from build123d import *

# Parameters (mm, degrees)
EXTRUDE_1_DEPTH             = 40
CUT_EXTRUDE_2_REACH         = 89.321
HOLE_WIZARD_M5_1_AT_2_COUNT = 2
HOLE_WIZARD_M5_1_AT_2_PITCH = 66.468037432
HOLE_WIZARD_M5_1_AT_3_COUNT = 2
HOLE_WIZARD_M5_1_AT_3_PITCH = 94
HOLE_WIZARD_M5_1_AT_4_COUNT = 2
HOLE_WIZARD_M5_1_AT_4_PITCH = 66.468037432
SKETCH_5_R                  = 17.5
CUT_EXTRUDE_3_DEPTH         = 10


with BuildPart() as part:
    # 草图1 → 拉伸1 (new, symmetric)
    with BuildSketch(Plane.XY):
        Polygon((-20, 0), (10, 0), (10, 85), (0, 85), (0, 10), (-20, 10), align=None)
    extrude(amount=EXTRUDE_1_DEPTH, both=True)

    # 草图2 → 拉伸2 (cut, up to next)
    with BuildSketch(Plane(origin=(0, 10, 0), x_dir=(1, 0, 0), z_dir=(0, 1, 0)), mode=Mode.PRIVATE) as cut_extrude_2_sk1:
        with BuildLine():
            Line((-13.5, 25), (-13.5, 15))
            ThreePointArc((-13.5, 15), (-10, 11.5), (-6.5, 15))
            Line((-6.5, 15), (-6.5, 25))
            ThreePointArc((-6.5, 25), (-10, 28.5), (-13.5, 25))
        make_face()
    cut_extrude_2_tool1 = extrude(cut_extrude_2_sk1.sketch, amount=-CUT_EXTRUDE_2_REACH, mode=Mode.PRIVATE) & part.part
    # 草图2 → 拉伸2 (cut, up to next)
    with BuildSketch(Plane(origin=(0, 10, 0), x_dir=(1, 0, 0), z_dir=(0, 1, 0)), mode=Mode.PRIVATE) as cut_extrude_2_sk2:
        with BuildLine():
            Line((-13.5, -15), (-13.5, -25))
            ThreePointArc((-13.5, -25), (-10, -28.5), (-6.5, -25))
            Line((-6.5, -25), (-6.5, -15))
            ThreePointArc((-6.5, -15), (-10, -11.5), (-13.5, -15))
        make_face()
    cut_extrude_2_tool2 = extrude(cut_extrude_2_sk2.sketch, amount=-CUT_EXTRUDE_2_REACH, mode=Mode.PRIVATE) & part.part
    add(cut_extrude_2_tool1.solids().sort_by_distance((-10, 10, -20))[0], mode=Mode.SUBTRACT)
    add(cut_extrude_2_tool2.solids().sort_by_distance((-10, 10, 20))[0], mode=Mode.SUBTRACT)

    # 草图3 → M5 螺纹孔1 (revolve, cut)
    with BuildSketch(Plane(origin=(0, 78.234018716, 33.234018716), x_dir=(0, 0, 1), z_dir=(0, 1, 0))):
        Polygon((0, 0), (0, 15.2618073), (2.1, 14), (2.1, 0), align=None)
    hole_wizard_m5_1 = revolve(axis=Axis((-6.35, 78.234018716, 33.234018716), (1, 0, 0)), mode=Mode.SUBTRACT)

    # M5 螺纹孔1 at 2: M5 螺纹孔1 ×2
    with Locations(*[(0, 0, -i * HOLE_WIZARD_M5_1_AT_2_PITCH) for i in range(1, HOLE_WIZARD_M5_1_AT_2_COUNT)]):
        add(hole_wizard_m5_1, mode=Mode.SUBTRACT)

    # M5 螺纹孔1 at 3: M5 螺纹孔1 ×2
    with Locations(*[Vector(0, -0.7071067811865464, -0.7071067811865487) * (i * HOLE_WIZARD_M5_1_AT_3_PITCH) for i in range(1, HOLE_WIZARD_M5_1_AT_3_COUNT)]):
        add(hole_wizard_m5_1, mode=Mode.SUBTRACT)

    # M5 螺纹孔1 at 4: M5 螺纹孔1 ×2
    with Locations(*[(0, -i * HOLE_WIZARD_M5_1_AT_4_PITCH, 0) for i in range(1, HOLE_WIZARD_M5_1_AT_4_COUNT)]):
        add(hole_wizard_m5_1, mode=Mode.SUBTRACT)

    # 草图5 → 拉伸3 (cut)
    with BuildSketch(Plane.ZY):
        with Locations(Location((0, 60, 0), (0, 0, 270))):
            Circle(SKETCH_5_R)
    extrude(amount=-CUT_EXTRUDE_3_DEPTH, mode=Mode.SUBTRACT)


solid = part.part
The model under review builds one solid part; all positions refer to its coordinate system, in mm. A direction names the side the tool comes from. Give positions to 0.01 mm unless a question says otherwise; leave off trailing zeros. Order: outer loops, then holes, each group sorted by start corner. A loop starts at its lowest first (then second) coordinate and runs counter-clockwise, first axis right, second up. Notation, with made-up numbers: M 62.25,-37.75 L 96.25,-37.75 A15 cw 96.25,-21.75 Z; hole C -33,-25.75 d4. An arc over 180 degrees is marked long. One line per question, with ' | ' between items. Start each with the question number.
1) Consider section B-B, the plane y = 6. Give the boundary of the cut face in (x, z).
2) Clearance check with flat-ended pins moving along their axes: P1, Ø10, axis at x = -12.5, z = 0, coming from the +Y side; P2, Ø5, axis at x = -0.5, z = 14, coming from the -Y side; P3, Ø5, axis at y = 39.5, z = 11, coming from the -X side. State where each tip first meets the part, or that it passes through.
3) Consider section C-C, the plane z = -23.5. Give the boundary of the cut face in (x, y).
4) Wall thickness on L1, parallel to Z at x = -10.25, y = 4; L2, parallel to Y at x = 8.5, z = -33.5; L3, parallel to Z at x = 2, y = 60: over which ranges is each line inside the solid? List them lowest first. Write a range as from..to.
5) For faces 5 (the face through (4.93, 76.152, -33.507)), 6 (the face through (-9.9, 5.1, 11.5)), 7 (the face through (0, 40, 1)), list the 3-axis set-ups (+Z, -Z, +X, -X, +Y, -Y) from which the entire face can be reached by the end or side of a thin tool; tool diameter is ignored.
6) Consider section A-A, the plane x = -10. Give the boundary of the cut face in (y, z), then the cut area to 3 significant figures.
7) Consider section D-D, the plane y = 60. Give the boundary of the cut face in (x, z).
8) Mouldability with a two-part tool opening along X and no side actions: class faces 1 (the face through (-20, 5, 1)), 2 (the face through (-6.5, 5, 20)), 3 (the face through (-10.1, 5.1, -11.5)), 4 (the face through (-5, 0, 1)) as pulls with the +X half, pulls with the -X half, needs draft (parallel to the pull), parting line crosses it, or undercut.
Found:
1) outline: M -20,-40 L 10,-40 L 10,40 L -20,40 Z; hole M -13.5,-25 A3.5 ccw -6.5,-25 L -6.5,-15 A3.5 ccw -13.5,-15 Z; hole M -13.5,15 A3.5 ccw -6.5,15 L -6.5,25 A3.5 ccw -13.5,25 Z
2) P1: stops at y = 10 | P2: stops at y = 0 | P3: stops at x = 0
3) outline: M -20,0 L -13.5,0 L -13.5,10 L -20,10 Z; M -6.5,0 L 10,0 L 10,85 L 0,85 L 0,10 L -6.5,10 Z
4) L1: z = -40..-28.49, -11.51..11.51, 28.49..40 | L2: y = 0..9.68, 13.85..76.15, 80.32..85 | L3: z = -40..-17.5, 17.5..40
5) face 5: +X, -X | face 6: +Y, -Y | face 7: +Z, -Z, -X, +Y
6) outline: M 0,-40 L 10,-40 L 10,-28.5 L 0,-28.5 Z; M 0,-11.5 L 10,-11.5 L 10,11.5 L 0,11.5 Z; M 0,28.5 L 10,28.5 L 10,40 L 0,40 Z | area: 460 mm²
7) outline: M 0,-40 L 10,-40 L 10,-17.5 L 0,-17.5 Z; M 0,17.5 L 10,17.5 L 10,40 L 0,40 Z
8) face 1: pulls with the -X half | face 2: undercut | face 3: undercut | face 4: needs draft
